Part model, mm, in its own coordinate system. A direction names the side the tool comes from. Coordinates: 2 decimals unless noted, no trailing zeros. Write each loop counter-clockwise with the first axis right and the second up, starting at its lowest first coordinate (ties: lowest second). Pieces come first, ordered by that corner, then holes. Notation, with made-up numbers: M 8,73 L 25,73 A14 cw 25,83 Z; hole C 84,-18 d9. An arc over 180 degrees is marked long. Use a Markdown table: item, result. Add a question column.
Q1. Slice it at A-A on x = 49. Write the cut outline in (y, z).
Q2. Slice it at D-D on y = -28.5. Write the cut outline in (x, z), then the cut area to 3 significant figures.
Q3. Slice it at C-C on y = 61. Write the cut outline in (x, z), then the cut area to 3 significant figures.
Q4. Tool access for faces 1 (the cylindrical face through (32.419, 64.794, 6.648)), 2 (the cylindrical face through (-31.5, -13.93, 5.27)): list every direction of +Z, -Z, +X, -X, +Y, -Y with a clear straight run to the whole face (end or side of a thin tool).
Q5. Slice it at B-B on z = 4.5. Write the cut outline in (x, y).
Q6. Wall check: L1, parallel to Y at x = -30, z = 2.75; L2, parallel to Y at x = -30, z = 6; L3, parallel to X at y = 60, z = 5. Give the ranges that are in metal, low to high. Write a range as from..to.
Q7. Pin check, flat tip, straight feed: pin 1 Ø7.5 at (x, y) = (49, 53) entering from +Z. Stop position of the tip, or through.
Q8. Mould opens along Y. For faces 3 (the cylindrical face through (-31.11, 62.01, 5.27)), 4 (the flat face through (-1, 67, 1)), 5 (the flat face through (-30, -16, 10.4)) say: released by +Y, released by -Y, zero draft, split by the parting line, or undercut.
from build123d import *

# Parameters (mm, degrees)
SKETCH001_W     = 126
SKETCH001_H     = 134
SKETCH001_R     = 2.4
PAD_DEPTH       = 3
SKETCH009_R     = 4.5
PAD005_DEPTH    = 7.4
SKETCH010_R     = 1.5
POCKET017_DEPTH = 10.401
CHAMFER015_SIZE = 1


with BuildPart() as part:
    # Sketch001 → Pad (new body)
    with BuildSketch(Plane.XY):
        Rectangle(SKETCH001_W, SKETCH001_H)
        with Locations((-49, 53)):
            Circle(SKETCH001_R, mode=Mode.SUBTRACT)
        with Locations((49, 53)):
            Circle(SKETCH001_R, mode=Mode.SUBTRACT)
        with Locations((-49, -53)):
            Circle(SKETCH001_R, mode=Mode.SUBTRACT)
        with Locations((49, -53)):
            Circle(SKETCH001_R, mode=Mode.SUBTRACT)
        with Locations((55, 37)):
            Circle(SKETCH001_R, mode=Mode.SUBTRACT)
        with Locations((-55, 37)):
            Circle(SKETCH001_R, mode=Mode.SUBTRACT)
        with Locations((-55, -37)):
            Circle(SKETCH001_R, mode=Mode.SUBTRACT)
        with Locations((55, -37)):
            Circle(SKETCH001_R, mode=Mode.SUBTRACT)
    extrude(amount=PAD_DEPTH)

    # Sketch009 (on Face14 of Pad) → Pad005 (join)
    with BuildSketch(Plane.XY.offset(3)):
        with Locations((-30, 61)):
            Circle(SKETCH009_R)
        with Locations((30, 61)):
            Circle(SKETCH009_R)
        with Locations((-30, -14)):
            Circle(SKETCH009_R)
        with Locations((30, -14)):
            Circle(SKETCH009_R)
    extrude(amount=PAD005_DEPTH)

    # Sketch010 (on Face22 of Pad005) → Pocket017 (cut, through all)
    with BuildSketch(Plane.XY.offset(10.4)):
        with Locations((-30, 61)):
            Circle(SKETCH010_R)
        with Locations((30, 61)):
            Circle(SKETCH010_R)
        with Locations((30, -14)):
            Circle(SKETCH010_R)
        with Locations((-30, -14)):
            Circle(SKETCH010_R)
    extrude(amount=-POCKET017_DEPTH, mode=Mode.SUBTRACT)

    # Chamfer015
    chamfer015_edges = [part.edges().sort_by_distance(p)[0] for p in [
        (-63, 0, 0),
        (63, 0, 0),
    ]]
    chamfer(chamfer015_edges, length=CHAMFER015_SIZE)


solid = part.part
Recorded:
| question | item | result |
|---|---|---|
| 1 | outline | M -67,0 L -55.4,0 L -55.4,3 L -67,3 Z; M -50.6,0 L 50.6,0 L 50.6,3 L -50.6,3 Z; M 55.4,0 L 67,0 L 67,3 L 55.4,3 Z |
| 2 | outline | M -63,1 L -62,0 L 62,0 L 63,1 L 63,3 L -63,3 Z |
| 2 | area | 377 mm² |
| 3 | outline | M -63,1 L -62,0 L -31.5,0 L -31.5,10.4 L -34.5,10.4 L -34.5,3 L -63,3 Z; M -28.5,0 L 28.5,0 L 28.5,10.4 L 25.5,10.4 L 25.5,3 L -25.5,3 L -25.5,10.4 L -28.5,10.4 Z; M 31.5,0 L 62,0 L 63,1 L 63,3 L 34.5,3 L 34.5,10.4 L 31.5,10.4 Z |
| 3 | area | 448 mm² |
| 4 | face 1 | +Z |
| 4 | face 2 | +Z, -Z |
| 5 | outline | C -30,-14 d9; C -30,61 d9; C 30,-14 d9; C 30,61 d9; hole C -30,-14 d3; hole C -30,61 d3; hole C 30,-14 d3; hole C 30,61 d3 |
| 6 | L1 | -67..-15.5, -12.5..59.5, 62.5..67 |
| 6 | L2 | -18.5..-15.5, -12.5..-9.5, 56.5..59.5, 62.5..65.5 |
| 6 | L3 | -34.39..-31.12, -28.88..-25.61, 25.61..28.88, 31.12..34.39 |
| 7 | pin 1 | z = 3 |
| 8 | face 3 | undercut |
| 8 | face 4 | released by +Y |
| 8 | face 5 | zero draft |
